Source: CAD feature listing. Evaluate the final solid. Frame: model axes, mm. Face numbers are marked on the shaded views. Coordinates: 2 decimals unless noted, no trailing zeros. Write each loop counter-clockwise with the first axis right and the second up, starting at its lowest first coordinate (ties: lowest second). Pieces come first, ordered by that corner, then holes. Notation, with made-up numbers: M -18,9 L 0,9 A28 ccw 0,45 Z; hole C 20.25,-24.5 d2. An arc over 180 degrees is marked long. One line per item, written item: value. Start each with the question number.
Item 1: Cut plane B-B, the plane y = 30. Output: boundary loops of the cut face in (x, z), then the cut area to 3 significant figures.
Item 2: Mould query, pull axis X, two halves, no side actions, for the marked faces 1 and 2. Classes: released by +X, released by -X, zero draft, split by the parting line, or undercut.
Item 3: Pin query (flat end, axial travel): P1, Ø3, axis at x = -15.5, y = -35.5, coming from the -Z side; P2, Ø1, axis at x = -36.5, y = 16.5, coming from the +Z side. Return the tip coordinate at first contact, or that it passes through.
Item 4: Cut plane A-A, the plane z = 2.75. Output: boundary loops of the cut face in (x, y).
Item 5: Ray query, L1, parallel to Z at x = 42, y = 9.5; L2, parallel to X at y = 3.5, z = 2.55; L3, parallel to X at y = -6, z = 3.05. Return the intervals inside material, ascending. Write a range as from..to.
```python
from build123d import *

# Parameters (mm, degrees)
F0_W     = 100.0000410745
F0_H     = 100
F1_DEPTH = 2
F6_COUNT = 3


with BuildPart() as f1:
    # F0 (on Top) → F1 (new body)
    with BuildSketch(Plane.XY):
        with Locations((2.05373e-05, 0)):
            Rectangle(F0_W, F0_H)
    extrude(amount=F1_DEPTH)

    # F2 (on Right) → F3 (revolve)
    with BuildSketch(Plane.YZ):
        with BuildLine():
            Line((16, 0), (24, 0))
            ThreePointArc((24, 0), (20, 4), (16, 0))
        make_face()
    revolve(axis=Axis((0, 0, 3.7722848356), (0, 0, -1)))

    # F4 (on Right) → F5 (revolve)
    with BuildSketch(Plane.YZ):
        with BuildLine():
            Line((40, 0), (44, 0))
            ThreePointArc((44, 0), (42.8284271247, 2.8284271247), (40, 4))
            Line((40, 4), (40, 0))
        make_face()
    f5 = revolve(axis=Axis((0, 40, 1.4672121033), (0, 0, -1)))

    # F6: F5 ×3 about axis
    f6_axis = Axis((0, 0, 3.7722848356), (0, 0, -1))
    for i in range(1, F6_COUNT):
        add(f5.rotate(f6_axis, i * 360 / F6_COUNT))


solid = f1.part
```
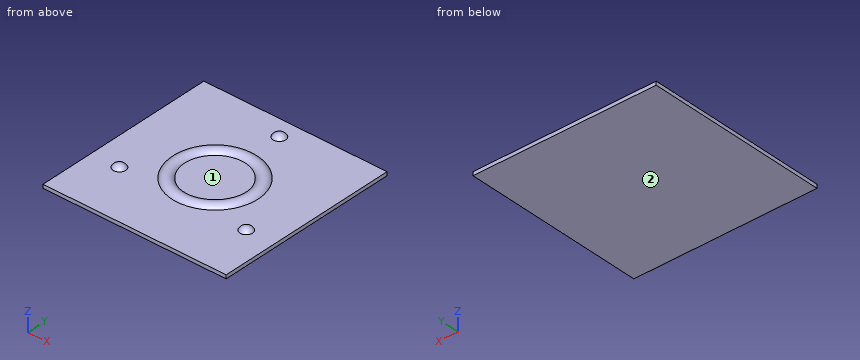
From the geometry:
1. outline: M -50,0 L 50,0 L 50,2 L -50,2 Z
1. area: 200 mm²
2. face 1: undercut
2. face 2: zero draft
3. P1: stops at z = 0
3. P2: stops at z = 2
4. outline: C -34.64,-20 d5.81; C 0,0 d45.81; C 0,40 d5.81; C 34.64,-20 d5.81; hole C 0,0 d34.19
5. L1: z = 0..2
5. L2: x = -22.81..-16.55, 16.55..22.81
5. L3: x = -21.78..-16.35, 16.35..21.78
